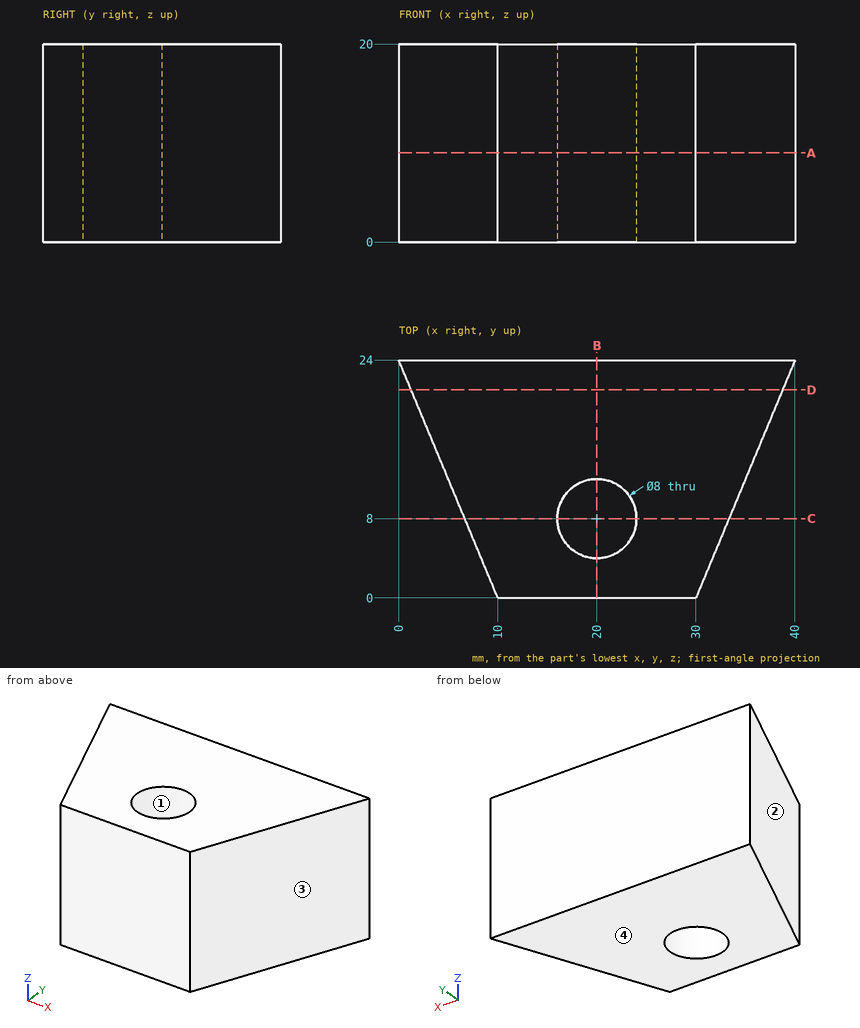
Study the drawing (mm; zero at the part's minimum x, y, z) and answer. Give positions to 0.01 mm unless a question says otherwise; leave off trailing zeros. Write each loop counter-clockwise with the first axis right and the second up, starting at its lowest first coordinate (ties: lowest second). Pieces come first, ordered by that corner, then holes. Notation, with made-up numbers: (42.25, 44) -> (73.25, 44) arc R22 cw to (73.25, 60) -> close; hole circle Ø4 at (37, 57.5). An arc over 180 degrees is marked (long way). Answer in a Markdown table with one row per item.
1) Each of these flat-tipped pins is pushed along its axis until it touches: pin 1 Ø5 at (y, z) = (7, 8.5) entering from +X; pin 2 Ø1.5 at (x, z) = (13.5, 6) entering from -Y; pin 3 Ø4 at (x, z) = (34.5, 16) entering from -Y; pin 4 Ø10 at (y, z) = (16, 17) entering from +X. Where does it stop, or does it pass through?
Results list:
| item | result |
|---|---|
| pin 1 | x = 33.96 |
| pin 2 | y = 0 |
| pin 3 | y = 6 |
| pin 4 | x = 38.75 |
2) Section D-D on y = 21 is taken. Give the vertices of the cut face in (x, z).
Results list:
| item | result |
|---|---|
| outline | (1.25, 0) -> (38.75, 0) -> (38.75, 20) -> (1.25, 20) -> close |
3) Determine the mould class of the marked faces 1, 2, 3 and 4 for opening direction X: released by +X, released by -X, zero draft, split by the parting line, or undercut.
Results list:
| item | result |
|---|---|
| face 1 | undercut |
| face 2 | released by -X |
| face 3 | released by +X |
| face 4 | zero draft |
4) Section A-A on z = 9 is taken. Give the vertices of the cut face in (x, y), plus the area to 3 significant figures.
Results list:
| item | result |
|---|---|
| outline | (0, 24) -> (10, 0) -> (30, 0) -> (40, 24) -> close; hole circle Ø8 at (20, 8) |
| area | 670 mm^2 |
5) Section C-C on y = 8 is taken. Give the vertices of the cut face in (x, z).
Results list:
| item | result |
|---|---|
| outline | (6.67, 0) -> (16, 0) -> (16, 20) -> (6.67, 20) -> close; (24, 0) -> (33.33, 0) -> (33.33, 20) -> (24, 20) -> close |
6) Straight lines are drawn through the part: line 1 (Y direction, x = 20, z = 14); line 2 (X direction, y = 8, z = 6.25); line 3 (X direction, y = 11.25, z = 16). For each, find the intervals that lie inside material, in ascending order. Write a range as [from, to].
Results list:
| item | result |
|---|---|
| line 1 | [0, 4], [12, 24] |
| line 2 | [6.67, 16], [24, 33.33] |
| line 3 | [5.31, 17.67], [22.33, 34.69] |
7) Section B-B on x = 20 is taken. Give the vertices of the cut face in (y, z), plus the area to 3 significant figures.
Results list:
| item | result |
|---|---|
| outline | (0, 0) -> (4, 0) -> (4, 20) -> (0, 20) -> close; (12, 0) -> (24, 0) -> (24, 20) -> (12, 20) -> close |
| area | 320 mm^2 |
